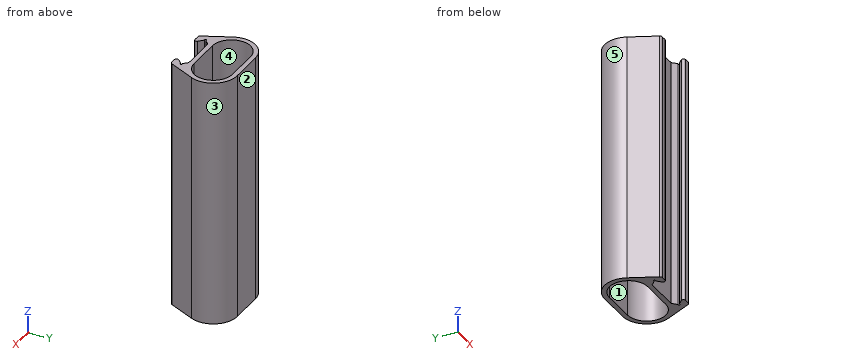
from build123d import *

# Parameters (mm, degrees)
F1_DEPTH = 123.825


with BuildPart() as f1:
    # F0 (on Top) → F1 (new body)
    with BuildSketch(Plane.XY):
        with BuildLine():
            ThreePointArc((-10.949447, -14.291553), (-11.803, -13.938), (-10.949447, -13.584447))
            Line((-10.949447, -13.584447), (-8.756901, -11.391901))
            Line((-8.756901, -11.391901), (8.769099, -11.391901))
            Line((8.769099, -11.391901), (10.955546, -13.578347))
            ThreePointArc((10.955546, -13.578347), (11.809099, -13.931901), (10.955546, -14.285454))
            Line((10.955546, -14.285454), (8.763, -16.478))
            ThreePointArc((8.763, -16.478), (8.546227, -17.56779), (9.470107, -18.185107))
            Line((9.470107, -18.185107), (12.033, -18.185107))
            ThreePointArc((12.033, -18.185107), (12.716208, -17.98568), (13.184849, -17.450031))
            Line((13.184849, -17.450031), (19.203687, -4.489717))
            ThreePointArc((19.203687, -4.489717), (18.440529, 6.948259), (8.388099, 12.458099))
            Line((8.388099, 12.458099), (-8.375901, 12.458099))
            ThreePointArc((-8.375901, 12.458099), (-18.425847, 6.95215), (-19.195375, -4.481341))
            Line((-19.195375, -4.481341), (-13.185263, -17.449139))
            ThreePointArc((-13.185263, -17.449139), (-12.716622, -17.985415), (-12.033, -18.185107))
            Line((-12.033, -18.185107), (-9.470107, -18.185107))
            ThreePointArc((-9.470107, -18.185107), (-8.546227, -17.56779), (-8.763, -16.478))
            Line((-8.763, -16.478), (-10.949447, -14.291553))
        make_face()
        with BuildLine():
            ThreePointArc((8.388099, 10.058099), (17.913099, 0.533099), (8.388099, -8.991901))
            Line((8.388099, -8.991901), (-8.375901, -8.991901))
            ThreePointArc((-8.375901, -8.991901), (-17.900901, 0.533099), (-8.375901, 10.058099))
            Line((-8.375901, 10.058099), (8.388099, 10.058099))
        make_face(mode=Mode.SUBTRACT)
    extrude(amount=F1_DEPTH)


solid = f1.part
Design review of the part built by this model. Coordinates are the model's own, in mm. Face numbers are marked on the shaded views. A direction names the side the tool comes from. Coordinates: 2 decimals unless noted, no trailing zeros. Loops run counter-clockwise (first coordinate to the right, second up) from the corner with the lowest first, then second, coordinate; pieces in that order, holes last. Notation, with made-up numbers: M 28,2 L 36,2 A30 ccw 36,34 Z; hole C 74.25,37.5 d3. An arc over 180 degrees is marked long. Answer as CSV lines item,"result".
Item 1: The part is to be moulded in two halves that separate along Y. For the marked faces 1, 2 and 3, say which applies: pulls with the +Y half, pulls with the -Y half, needs draft (parallel to the pull), parting line crosses it, or undercut.
Answer list:
face 1,"undercut"
face 2,"pulls with the +Y half"
face 3,"parting line crosses it"
Item 2: Machinability: for the marked faces 4 and 5, which of the approach directions +Z, -Z, +X, -X, +Y, -Y give a long, thin tool a straight path to every point of the face, cutting with its end or side? Answer none if there is none.
Answer list:
face 4,"+Z, -Z"
face 5,"+Z, -Z, -X"
Item 3: For probe 1 along Y at (x, z) = (-1, 85); probe 2 along Y at (x, z) = (11.5, 48); probe 3 along X at (y, z) = (0, 30), list the stretches that pass through material, from the lowest coordinate up.
Answer list:
probe 1,"-11.39 to -8.99, 10.06 to 12.46"
probe 2,"-18.19 to -14.39, -13.47 to -8.47, 9.54 to 12.04"
probe 3,"-20.29 to -17.89, 17.9 to 20.3"
Item 4: For P1, Ø10, axis at x = 7, y = 5, coming from the +Z side; P2, Ø8, axis at y = -9, z = 91, coming from the +X side; P3, Ø8.5, axis at x = -3.5, z = 70, coming from the -Y side; P4, Ø3, axis at x = 15.5, z = 26.5, coming from the -Y side, all flat-tipped, find the tip position at first contact; note any pin that passes through.
Answer list:
P1,"through"
P2,"x = 18.97"
P3,"y = -11.39"
P4,"y = -15.69"
Item 5: Add section A-A on x = 5. State the section outline as (y, z) points (3 decimals).
Answer list:
outline,"M -11.392,0 L -8.992,0 L -8.992,123.825 L -11.392,123.825 Z; M 10.058,0 L 12.458,0 L 12.458,123.825 L 10.058,123.825 Z"
Item 6: Add section C-C on z = 39. State the section outline as (x, y) points (3 decimals), plus the area to 3 significant figures.
Answer list:
outline,"M -19.195,-4.481 L -13.185,-17.449 A1.27 ccw -12.033,-18.185 L -9.47,-18.185 A1 ccw -8.763,-16.478 L -10.949,-14.292 A0.5 cw long -10.949,-13.584 L -8.757,-11.392 L 8.769,-11.392 L 10.956,-13.578 A0.5 cw long 10.956,-14.285 L 8.763,-16.478 A1 ccw 9.47,-18.185 L 12.033,-18.185 A1.27 ccw 13.185,-17.45 L 19.204,-4.49 A11.925 ccw 8.388,12.458 L -8.376,12.458 A11.925 ccw Z; hole M -8.376,-8.992 L 8.388,-8.992 A9.525 ccw 8.388,10.058 L -8.376,10.058 A9.525 ccw Z"
area,"325 mm²"
Item 7: Add section B-B on y = -2. State the section outline as (x, z) points (3 decimals).
Answer list:
outline,"M -20.029,0 L -17.558,0 L -17.558,123.825 L -20.029,123.825 Z; M 17.57,0 L 20.041,0 L 20.041,123.825 L 17.57,123.825 Z"
